from build123d import *

# Parameters (mm, degrees)
CYLINDER014005899_R     = 7
CYLINDER014005899_DEPTH = 1
TUBE005_R               = 8
TUBE005_R_2             = 4.2
TUBE005_DEPTH           = 4.5


with BuildPart() as obj1:
    # Cylinder014005899 → Cylinder014005899 (new body)
    with BuildSketch(Plane.XY):
        Circle(CYLINDER014005899_R)
    extrude(amount=CYLINDER014005899_DEPTH)


with BuildPart() as ring001:
    # Tube005 → Tube005 (new body)
    with BuildSketch(Plane.XY):
        Circle(TUBE005_R)
        Circle(TUBE005_R_2, mode=Mode.SUBTRACT)
    extrude(amount=TUBE005_DEPTH)

    # Cut009003003009003003003003: cut obj1
    add(obj1.part, mode=Mode.SUBTRACT)


solid = ring001.part
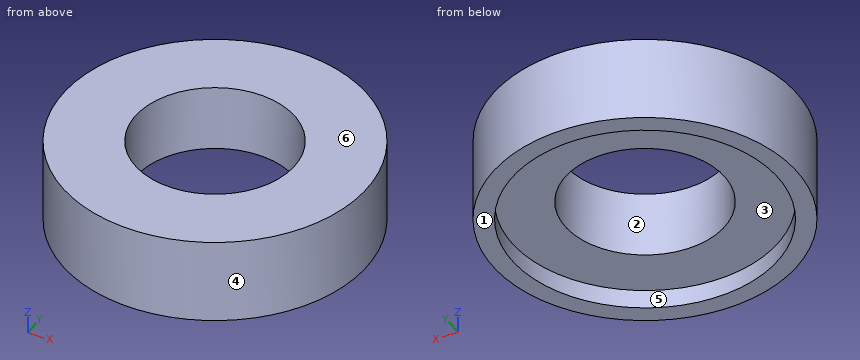
Input: part model. Units: mm. Frame: model coordinates. Face numbers are marked on the shaded views. A direction names the side the tool comes from. Round coordinates to 2 decimals unless told otherwise and drop trailing zeros. Order: outer loops, then holes, each group sorted by start corner. A loop starts at its lowest first (then second) coordinate and runs counter-clockwise, first axis right, second up. Notation, with made-up numbers: (70.25, -15) - (101.25, -15) arc R22 ccw to (101.25, -2) - close; hole circle Ø4 at (48, 31.5). An arc over 180 degrees is marked (long way). Use a Markdown table: item, result.
1. Section C-C on z = 3.45. Return the cut outline in (x, y), then the cut area to 3 significant figures.
Evaluation:
| item | result |
|---|---|
| outline | circle Ø16 at (0, 0); hole circle Ø8.4 at (0, 0) |
| area | 146 mm^2 |
2. First-contact query: pin 1 (5 mm diameter, centred on x = 0, y = 0, fed in from -Z); pin 2 (7 mm diameter, centred on x = -2.5, y = 0.5, fed in from -Z). Flat tips, straight axial feed; report the tip coordinate or a pass-through.
Evaluation:
| item | result |
|---|---|
| pin 1 | through |
| pin 2 | z = 1 |
3. Access query for the marked faces 5 and 6. Directions: +Z, -Z, +X, -X, +Y, -Y. A direction counts if a zero-diameter tool reaches every point of the face in a straight line with its end or side. Return the directions, or none.
Evaluation:
| item | result |
|---|---|
| face 5 | -Z |
| face 6 | +Z, +X, -X, +Y, -Y |
4. Section A-A on y = 0. Return the cut outline in (x, z), then the cut area to 3 significant figures.
Evaluation:
| item | result |
|---|---|
| outline | (-8, 0) - (-7, 0) - (-7, 1) - (-4.2, 1) - (-4.2, 4.5) - (-8, 4.5) - close; (4.2, 1) - (7, 1) - (7, 0) - (8, 0) - (8, 4.5) - (4.2, 4.5) - close |
| area | 28.6 mm^2 |
5. Material intervals for probe 1 along Y at (x, z) = (0, 0.6); probe 2 along Y at (x, z) = (0, 2.1); probe 3 along X at (y, z) = (-1.5, 4), sorted ascending.
Evaluation:
| item | result |
|---|---|
| probe 1 | -8 to -7, 7 to 8 |
| probe 2 | -8 to -4.2, 4.2 to 8 |
| probe 3 | -7.86 to -3.92, 3.92 to 7.86 |
6. Section D-D on y = 6.75. Return the cut outline in (x, z), then the cut area to 3 significant figures.
Evaluation:
| item | result |
|---|---|
| outline | (-4.29, 0) - (-1.85, 0) - (-1.85, 1) - (1.85, 1) - (1.85, 0) - (4.29, 0) - (4.29, 4.5) - (-4.29, 4.5) - close |
| area | 34.9 mm^2 |
7. Mould query, pull axis Y, two halves, no side actions, for the marked faces 1, 2, 3 and 4. Classes: +Y half, -Y half, draft (parallel to the pull), parting line (faces both ways), or undercut.
Evaluation:
| item | result |
|---|---|
| face 1 | draft |
| face 2 | undercut |
| face 3 | undercut |
| face 4 | parting line |
